Could you check a few things on this model? Use its own coordinates, in mm. A direction names the side the tool comes from. Give positions to 0.01 mm unless a question says otherwise; leave off trailing zeros. Write each loop counter-clockwise with the first axis right and the second up, starting at its lowest first coordinate (ties: lowest second). Pieces come first, ordered by that corner, then holes. Notation, with made-up numbers: (76, 73) - (101, 73) arc R18 ccw to (101, 82) - close; hole circle Ø3 at (-17.75, 35.5). An arc over 180 degrees is marked (long way). Answer in a Markdown table with one row per item.
from build123d import *

# Parameters (mm, degrees)
EXTRUDE_1_DEPTH     = 20
SKETCH_3_R          = 2.5
CUT_EXTRUDE_1_DEPTH = 20
SKETCH_9_W          = 6.520982116
SKETCH_9_H          = 12.021095894
CUT_EXTRUDE_4_DEPTH = 5
SKETCH_10_R         = 1
CUT_EXTRUDE_6_DEPTH = 7


with BuildPart() as part:
    # 草图1 → 凸台-拉伸1 (new body)
    with BuildSketch(Plane.XY):
        with BuildLine():
            Line((0, 20), (0, 10))
            ThreePointArc((0, 10), (-10, 0), (0, -10))
            Line((0, -10), (0, -20))
            Line((0, -20), (-20, -20))
            Line((-20, -20), (-20, 20))
            Line((-20, 20), (0, 20))
        make_face()
    extrude(amount=EXTRUDE_1_DEPTH)

    # 草图3 → 切除-拉伸1 (cut)
    with BuildSketch(Plane(origin=(0, 0, 0), x_dir=(0, 0, -1), z_dir=(1, 0, 0))):
        with Locations((-10, 15)):
            Circle(SKETCH_3_R)
        with Locations((-10, -15)):
            Circle(SKETCH_3_R)
    extrude(amount=-CUT_EXTRUDE_1_DEPTH, mode=Mode.SUBTRACT)

    # 草图9 → 切除-拉伸4 (cut)
    with BuildSketch(Plane(origin=(-20, 0, 0), x_dir=(0, 0, -1), z_dir=(1, 0, 0))):
        with Locations((-10, 0)):
            Rectangle(SKETCH_9_W, SKETCH_9_H)
    extrude(amount=CUT_EXTRUDE_4_DEPTH, mode=Mode.SUBTRACT)

    # 草图10 → 切除-拉伸6 (cut)
    with BuildSketch(Plane.XY):
        with Locations((-16.577606786, 0)):
            Circle(SKETCH_10_R)
    extrude(amount=CUT_EXTRUDE_6_DEPTH, mode=Mode.SUBTRACT)


solid = part.part
1) Imagine slicing it at C-C (z = 5.5). List the corners of the cut face in (x, y) for me, then the cut area to 3 significant figures.
Check values:
| item | result |
|---|---|
| outline | (-20, -20) - (0, -20) - (0, -10) arc R10 cw to (0, 10) - (0, 20) - (-20, 20) - close; hole circle Ø2 at (-16.58, 0) |
| area | 640 mm2 |
2) We'd pull the mould along Y, two halves only. Please class faces 3 (the face through (-12, 0, 20)), 4 (the face through (-10, 20, 10)), 5 (the face through (-17.577, 0.044, 3.323)): +Y half, -Y half, draft (parallel to the pull), parting line (faces both ways), or undercut.
Check values:
| item | result |
|---|---|
| face 3 | draft |
| face 4 | +Y half |
| face 5 | undercut |
3) If I drill on line 1 (Y direction, x = -13, z = 10); line 2 (X direction, y = 0, z = 2.75); line 3 (Y direction, x = -8.75, z = 10), over which ranges is the centre line in solid material (lowest first)?
Check values:
| item | result |
|---|---|
| line 1 | y = -20 to -17.5, -12.5 to 12.5, 17.5 to 20 |
| line 2 | x = -20 to -17.58, -15.58 to -10 |
| line 3 | y = -20 to -17.5, -12.5 to -4.84, 4.84 to 12.5, 17.5 to 20 |
4) On a 3-axis mill with a long thin cutter (end or side, diameter ignored), from which of +Z, -Z, +X, -X, +Y, -Y can I reach the whole of each face in a straight line? I mean faces 1 (the face through (-9.9, 13.5, 12)), 2 (the face through (-18, 0, 13.26)). Say none if no direction works.
Check values:
| item | result |
|---|---|
| face 1 | +X, -X |
| face 2 | -X |
5) Imagine slicing it at B-B (y = 15). List the corners of the cut face in (x, z) for me, then the cut area to 3 significant figures.
Check values:
| item | result |
|---|---|
| outline | (-20, 0) - (0, 0) - (0, 7.5) - (-20, 7.5) - close; (-20, 12.5) - (0, 12.5) - (0, 20) - (-20, 20) - close |
| area | 300 mm2 |
6) Will these pins go through, and if not, where does the flat tip stop? P1, Ø4, axis at y = -15, z = 10, coming from the +X side; P2, Ø7, axis at y = 1, z = 9.5, coming from the -X side.
Check values:
| item | result |
|---|---|
| P1 | passes through |
| P2 | stops at x = -20 |
7) Imagine slicing it at A-A (x = -6). List the corners of the cut face in (y, z) for me, then the cut area to 3 significant figures.
Check values:
| item | result |
|---|---|
| outline | (-20, 0) - (-8, 0) - (-8, 20) - (-20, 20) - close; (8, 0) - (20, 0) - (20, 20) - (8, 20) - close; hole circle Ø5 at (-15, 10); hole circle Ø5 at (15, 10) |
| area | 441 mm2 |
8) Imagine slicing it at D-D (z = 10). List the corners of the cut face in (x, y) for me.
Check values:
| item | result |
|---|---|
| outline | (-20, -20) - (0, -20) - (0, -17.5) - (-20, -17.5) - close; (-20, -12.5) - (0, -12.5) - (0, -10) arc R10 cw to (0, 10) - (0, 12.5) - (-20, 12.5) - (-20, 6.01) - (-15, 6.01) - (-15, -6.01) - (-20, -6.01) - close; (-20, 17.5) - (0, 17.5) - (0, 20) - (-20, 20) - close |
